```python
from build123d import *

# Parameters (mm, degrees)
BOSS_EXTRU_1_DEPTH       = 5
ESQUISSE6_R              = 34.85
ESQUISSE6_R_2            = 30
BOSS_EXTRU_6_DEPTH       = 7
BOSS_EXTRU_9_DEPTH       = 18
ENL_V_MAT_EXTRU_10_REACH = 84.676
ESQUISSE21_R             = 2.5
ESQUISSE22_R             = 4
ENL_V_MAT_EXTRU_11_DEPTH = 1
CONG_1_R                 = 20
CONG_2_R                 = 5
ESQUISSE11_W             = 20.2
ESQUISSE11_H             = 20.2
ENL_V_MAT_EXTRU_2_DEPTH  = 25
ESQUISSE12_R             = 2.65
ENL_V_MAT_EXTRU_3_DEPTH  = 81.451974996
ENL_V_START              = -5
ESQUISSE13_R             = 4.5
ENL_V_MAT_EXTRU_4_DEPTH  = 76.451974996
ENL_V_MAT_EXTRU_5_DEPTH  = 2
ENL_V_MAT_EXTRU_7_DEPTH  = 3
ESQUISSE19_R             = 1.65
ENL_V_MAT_EXTRU_8_DEPTH  = 82.890843677
ENL_V_MAT_EXTRU_9_DEPTH  = 1


with BuildPart() as part:
    # Esquisse1 → Boss.-Extru.1 (new body)
    with BuildSketch(Plane.XY):
        with BuildLine():
            Line((-45.620718977, 15), (-70, 15))
            Line((-70, 15), (-70, -15))
            Line((-70, -15), (-45.620718977, -15))
            ThreePointArc((-45.620718977, -15), (-36.774201608, -17.062911874), (-29.752642811, -22.826086957))
            ThreePointArc((-29.752642811, -22.826086957), (37.5, 0), (-29.752642811, 22.826086957))
            ThreePointArc((-29.752642811, 22.826086957), (-36.774201608, 17.062911874), (-45.620718977, 15))
        make_face()
    extrude(amount=BOSS_EXTRU_1_DEPTH)

    # Esquisse6 → Boss.-Extru.6 (add)
    with BuildSketch(Plane.XY.offset(5)):
        Circle(ESQUISSE6_R)
        Circle(ESQUISSE6_R_2, mode=Mode.SUBTRACT)
    extrude(amount=BOSS_EXTRU_6_DEPTH)

    # Esquisse8 → Boss.-Extru.9 (add)
    with BuildSketch(Plane.XY.offset(5)):
        with BuildLine():
            Line((-70, -15), (-70, 15))
            Line((-70, 15), (-43.874821937, 15))
            ThreePointArc((-43.874821937, 15), (-39.966142137, 13.118047822), (-38.999841722, 8.888888889))
            ThreePointArc((-38.999841722, 8.888888889), (-40, 0), (-38.999841722, -8.888888889))
            ThreePointArc((-38.999841722, -8.888888889), (-39.966142137, -13.118047822), (-43.874821937, -15))
            Line((-43.874821937, -15), (-70, -15))
        make_face()
    extrude(amount=BOSS_EXTRU_9_DEPTH)

    # Esquisse21 → Enlèv. mat.-Extru.10 (cut, up to next)
    with BuildSketch(Plane(origin=(0, 0, 0), x_dir=(-1, 0, 0), z_dir=(0, 0, -1)), mode=Mode.PRIVATE) as enl_v_mat_extru_10_sk1:
        with Locations((-19, 0)):
            Circle(ESQUISSE21_R)
    enl_v_mat_extru_10_tool1 = extrude(enl_v_mat_extru_10_sk1.sketch, amount=-ENL_V_MAT_EXTRU_10_REACH, mode=Mode.PRIVATE) & part.part
    # Esquisse21 → Enlèv. mat.-Extru.10 (cut, up to next)
    with BuildSketch(Plane(origin=(0, 0, 0), x_dir=(-1, 0, 0), z_dir=(0, 0, -1)), mode=Mode.PRIVATE) as enl_v_mat_extru_10_sk2:
        with Locations((19, 0)):
            Circle(ESQUISSE21_R)
    enl_v_mat_extru_10_tool2 = extrude(enl_v_mat_extru_10_sk2.sketch, amount=-ENL_V_MAT_EXTRU_10_REACH, mode=Mode.PRIVATE) & part.part
    add(enl_v_mat_extru_10_tool1.solids().sort_by_distance((19, 0, 0))[0], mode=Mode.SUBTRACT)
    add(enl_v_mat_extru_10_tool2.solids().sort_by_distance((-19, 0, 0))[0], mode=Mode.SUBTRACT)

    # Esquisse22 → Enlèv. mat.-Extru.11 (cut)
    with BuildSketch(Plane(origin=(0, 0, 0), x_dir=(-1, 0, 0), z_dir=(0, 0, -1))):
        with Locations((-19, 0)):
            Circle(ESQUISSE22_R)
        with Locations((19, 0)):
            Circle(ESQUISSE22_R)
    extrude(amount=-ENL_V_MAT_EXTRU_11_DEPTH, mode=Mode.SUBTRACT)

    # Congé1
    cong_1_edges = [part.edges().sort_by_distance(p)[0] for p in [
        (-70, 0, 0),
    ]]
    fillet(cong_1_edges, radius=CONG_1_R)

    # Congé2
    cong_2_edges = [part.edges().sort_by_distance(p)[0] for p in [
        (-47.810359489, -15, 0),
        (-36.774201608, -17.062911874, 0),
        (37.5, 0, 0),
        (-36.774201608, 17.062911874, 0),
        (-47.810359489, 15, 0),
        (-64.142135624, 15, 5.857864376),
        (-64.142135624, -15, 5.857864376),
        (-70, -15, 21.5),
        (-70, 15, 21.5),
    ]]
    fillet(cong_2_edges, radius=CONG_2_R - 0.0001)  # a hair under: the kernel refuses the full size

    # Esquisse11 → Enlèv. mat.-Extru.2 (cut)
    with BuildSketch(Plane.ZY.offset(70)):
        with Locations((23, 0)):
            Rectangle(ESQUISSE11_W, ESQUISSE11_H)
    extrude(amount=-ENL_V_MAT_EXTRU_2_DEPTH, mode=Mode.SUBTRACT)

    # Esquisse12 → Enlèv. mat.-Extru.3 (cut, through all)
    with BuildSketch(Plane.XY.offset(12.9)):
        with Locations((-51.5, 0)):
            Circle(ESQUISSE12_R)
        with Locations((-63.5, 0)):
            Circle(ESQUISSE12_R)
    extrude(amount=-ENL_V_MAT_EXTRU_3_DEPTH, mode=Mode.SUBTRACT)

    # Esquisse13 → Enlèv. mat.-Extru.4 (cut, through all)
    with BuildSketch(Plane.XY.offset(12.9).offset(ENL_V_START)):
        with Locations((-51.5, 0)):
            Circle(ESQUISSE13_R)
        with Locations((-63.5, 0)):
            Circle(ESQUISSE13_R)
    extrude(amount=-ENL_V_MAT_EXTRU_4_DEPTH, mode=Mode.SUBTRACT)

    # Esquisse14 → Enlèv. mat.-Extru.5 (cut)
    with BuildSketch(Plane.XY.offset(5)):
        with BuildLine():
            Line((-5.5, 10.5), (5.5, 10.5))
            ThreePointArc((5.5, 10.5), (9.035533906, 9.035533906), (10.5, 5.5))
            Line((10.5, 5.5), (10.5, -5.5))
            ThreePointArc((10.5, -5.5), (9.035533906, -9.035533906), (5.5, -10.5))
            Line((5.5, -10.5), (-5.5, -10.5))
            ThreePointArc((-5.5, -10.5), (-9.035533906, -9.035533906), (-10.5, -5.5))
            Line((-10.5, -5.5), (-10.5, 5.5))
            ThreePointArc((-10.5, 5.5), (-9.035533906, 9.035533906), (-5.5, 10.5))
        make_face()
    extrude(amount=-ENL_V_MAT_EXTRU_5_DEPTH, mode=Mode.SUBTRACT)

    # Esquisse17 → Enlèv. mat.-Extru.7 (cut)
    with BuildSketch(Plane(origin=(0, 0, 0), x_dir=(-1, 0, 0), z_dir=(0, 0, -1))):
        with BuildLine():
            Line((-5, -19.5), (-5, -15.5))
            ThreePointArc((-5, -15.5), (-5.878679656, -13.378679656), (-8, -12.5))
            Line((-8, -12.5), (-9.5, -12.5))
            ThreePointArc((-9.5, -12.5), (-11.621320344, -11.621320344), (-12.5, -9.5))
            Line((-12.5, -9.5), (-12.5, 9.5))
            ThreePointArc((-12.5, 9.5), (-11.621320344, 11.621320344), (-9.5, 12.5))
            Line((-9.5, 12.5), (-8, 12.5))
            ThreePointArc((-8, 12.5), (-5.878679656, 13.378679656), (-5, 15.5))
            Line((-5, 15.5), (-5, 19.5))
            ThreePointArc((-5, 19.5), (-4.121320344, 21.621320344), (-2, 22.5))
            Line((-2, 22.5), (2, 22.5))
            ThreePointArc((2, 22.5), (4.121320344, 21.621320344), (5, 19.5))
            Line((5, 19.5), (5, 15.5))
            ThreePointArc((5, 15.5), (5.878679656, 13.378679656), (8, 12.5))
            Line((8, 12.5), (9.5, 12.5))
            ThreePointArc((9.5, 12.5), (11.621320344, 11.621320344), (12.5, 9.5))
            Line((12.5, 9.5), (12.5, -9.5))
            ThreePointArc((12.5, -9.5), (11.621320344, -11.621320344), (9.5, -12.5))
            Line((9.5, -12.5), (8, -12.5))
            ThreePointArc((8, -12.5), (5.878679656, -13.378679656), (5, -15.5))
            Line((5, -15.5), (5, -19.5))
            ThreePointArc((5, -19.5), (4.121320344, -21.621320344), (2, -22.5))
            Line((2, -22.5), (-2, -22.5))
            ThreePointArc((-2, -22.5), (-4.121320344, -21.621320344), (-5, -19.5))
        make_face()
    extrude(amount=-ENL_V_MAT_EXTRU_7_DEPTH, mode=Mode.SUBTRACT)

    # Esquisse19 → Enlèv. mat.-Extru.8 (cut, through all)
    with BuildSketch(Plane(origin=(0, 0, 3), x_dir=(-1, 0, 0), z_dir=(0, 0, -1))):
        with Locations((0, 17.5)):
            Circle(ESQUISSE19_R)
        with Locations((0, -17.5)):
            Circle(ESQUISSE19_R)
    extrude(amount=-ENL_V_MAT_EXTRU_8_DEPTH, mode=Mode.SUBTRACT)

    # Esquisse20 → Enlèv. mat.-Extru.9 (cut)
    with BuildSketch(Plane.XY.offset(5)):
        Polygon((0, -14.035898385), (-3, -15.767949192), (-3, -19.232050808), (0, -20.964101615), (3, -19.232050808), (3, -15.767949192), align=None)
        Polygon((0, 14.035898385), (3, 15.767949192), (3, 19.232050808), (0, 20.964101615), (-3, 19.232050808), (-3, 15.767949192), align=None)
    extrude(amount=-ENL_V_MAT_EXTRU_9_DEPTH, mode=Mode.SUBTRACT)


solid = part.part
```
The listing builds one solid part. Answer for the finished solid, in the listing's coordinates (mm). A direction names the side the tool comes from. Give positions to 0.01 mm unless a question says otherwise; leave off trailing zeros. One line per item, written item: value.
Q1. Find the intervals of material crossed by line 1 (Y direction, x = -60.5, z = 21.5); line 2 (Y direction, x = -51.5, z = 9.2); line 3 (X direction, y = -7.5, z = 11.25), in increasing order. Write a range as from..to.
Working result:
line 1: y = -15..-10.1, 10.1..15
line 2: y = -15..-2.65, 2.65..15
line 3: x = -67.98..-39.29, -34.03..-29.05, 29.05..34.03
Q2. For faces 1 (the face through (0, -22.5, 1)), 2 (the face through (15.3, 26, 12)), 3 (the face through (-35, 0.2, 5)), determine the directions among +Z, -Z, +X, -X, +Y, -Y from which every point of the face is accessible in a straight line to the end or side of a thin tool.
Working result:
face 1: -Z
face 2: +Z, +X, +Y, -Y
face 3: +Z
Q3. Flat-ended cylindrical pins translate along their axes: P1, Ø2.5, axis at y = 18, z = 1.5, coming from the +X side; P2, Ø8, axis at x = 26.5, z = 18, coming from the +Y side; P3, Ø0.6, axis at x = -2, z = 4, coming from the -Y side; P4, Ø0.6, axis at y = 1, z = 4, coming from the -X side. Find the tip coordinate at first contact, or state that the pin passes through.
Working result:
P1: stops at x = 32.54
P2: passes through
P3: stops at y = -37.4
P4: stops at x = -59.19
Q4. A cutting plane is placed at A-A on y = 0. Give the number of separate pieces and of enclosed holes in the cut face, then the cut area to 3 significant figures.
Working result:
separate pieces: 6
enclosed holes: 0
area: 486 mm^2
Q5. Determine the mould class of faces 4 (the face through (-48, -14, 2)), 5 (the face through (13, 0, 5)), 6 (the face through (-18, 8, 0)) for opening direction Y: +Y half, -Y half, draft (parallel to the pull), parting line (faces both ways), or undercut.
Working result:
face 4: -Y half
face 5: undercut
face 6: draft
